from build123d import *

# Parameters (mm, degrees)
F1_DEPTH = 50.8


with BuildPart() as f1:
    # F0 (on Right) → F1 (new body)
    with BuildSketch(Plane.YZ):
        with BuildLine():
            ThreePointArc((38.1, 31.75), (36.240128, 36.240128), (31.75, 38.1))
            Line((31.75, 38.1), (12.7, 38.1))
            ThreePointArc((12.7, 38.1), (8.209872, 36.240128), (6.35, 31.75))
            Line((6.35, 31.75), (6.35, 20.128599))
            ThreePointArc((6.35, 20.128599), (6.851557, 18.393731), (8.201481, 17.194133))
            ThreePointArc((8.201481, 17.194133), (0, -19.05), (-8.201481, 17.194133))
            ThreePointArc((-8.201481, 17.194133), (-6.851557, 18.393731), (-6.35, 20.128599))
            Line((-6.35, 20.128599), (-6.35, 31.75))
            ThreePointArc((-6.35, 31.75), (-8.209872, 36.240128), (-12.7, 38.1))
            Line((-12.7, 38.1), (-31.75, 38.1))
            ThreePointArc((-31.75, 38.1), (-36.240128, 36.240128), (-38.1, 31.75))
            Line((-38.1, 31.75), (-38.1, -31.75))
            ThreePointArc((-38.1, -31.75), (-36.240128, -36.240128), (-31.75, -38.1))
            Line((-31.75, -38.1), (31.75, -38.1))
            ThreePointArc((31.75, -38.1), (36.240128, -36.240128), (38.1, -31.75))
            Line((38.1, -31.75), (38.1, 31.75))
        make_face()
    extrude(amount=F1_DEPTH)


solid = f1.part
Source: CAD feature listing. Evaluate the final solid. Frame: model axes, mm. A direction names the side the tool comes from. Round coordinates to 2 decimals unless told otherwise and drop trailing zeros. Loops run counter-clockwise (first coordinate to the right, second up) from the corner with the lowest first, then second, coordinate; pieces in that order, holes last. Notation, with made-up numbers: M -32,59 L 14,59 A9 ccw 14,65 Z; hole C -31.75,-35 d2. An arc over 180 degrees is marked long. Return JSON: item names as keys, results as strings. Group by question number.
1. Section query D-D on y = 0. Output: boundary loops of the cut face in (x, z).
2. Section query A-A on z = 0. Output: boundary loops of the cut face in (x, y), and give its area (3 significant figures).
3. Section query C-C on y = -16. Output: boundary loops of the cut face in (x, z).
4. Section query B-B on x = 22.5. Output: boundary loops of the cut face in (y, z), and give its area (3 significant figures).
5. Material intervals for line 1 along Y through (x, z) = (26, 0); line 2 along Z through (x, y) = (15, -15); line 3 along Z through (x, y) = (12, 13), sorted ascending. Write a range as from..to.
6. Pin query (flat end, axial travel): pin 1 (5 mm diameter, centred on x = 22, y = -8.5, fed in from +Z); pin 2 (12 mm diameter, centred on y = -23, z = 4, fed in from -X). Return the tip coordinate at first contact, or that it passes through.
7. Mould query, pull axis Y, two halves, no side actions, for faces 1 (the face through (25, 22, 38.1)), 2 (the face through (25, -38.1, 0)), 3 (the face through (25.04, 36.29, 36.19)), 4 (the face through (25.044, 0.719, -19.036)). Classes: released by +Y, released by -Y, zero draft, split by the parting line, or undercut.
8. Reachability of faces 5 (the face through (25.044, -6.865, 18.372)), 6 (the face through (25.04, 8.26, 36.29)), 7 (the face through (25.04, -36.19, 36.29)) from +Z, -Z, +X, -X, +Y, -Y: full face, straight path, thin tool, end or side. Return the list, or none.
Checks:
{
 "1": {"outline": "M 0,-38.1 L 50.8,-38.1 L 50.8,-19.05 L 0,-19.05 Z"},
 "2": {"outline": "M 0,-38.1 L 50.8,-38.1 L 50.8,-19.05 L 0,-19.05 Z; M 0,19.05 L 50.8,19.05 L 50.8,38.1 L 0,38.1 Z", "area": "1,940 mm²"},
 "3": {"outline": "M 0,-38.1 L 50.8,-38.1 L 50.8,-10.34 L 0,-10.34 Z; M 0,10.34 L 50.8,10.34 L 50.8,38.1 L 0,38.1 Z"},
 "4": {"outline": "M -38.1,-31.75 A6.35 ccw -31.75,-38.1 L 31.75,-38.1 A6.35 ccw 38.1,-31.75 L 38.1,31.75 A6.35 ccw 31.75,38.1 L 12.7,38.1 A6.35 ccw 6.35,31.75 L 6.35,20.13 A3.25 ccw 8.2,17.19 A19.05 cw long -8.2,17.19 A3.25 ccw -6.35,20.13 L -6.35,31.75 A6.35 ccw -12.7,38.1 L -31.75,38.1 A6.35 ccw -38.1,31.75 Z", "area": "4,370 mm²"},
 "5": {"line 1": "y = -38.1..-19.05, 19.05..38.1", "line 2": "z = -38.1..-11.74, 11.74..38.1", "line 3": "z = -38.1..-13.92, 13.92..38.1"},
 "6": {"pin 1": "stops at z = 37.87", "pin 2": "stops at x = 0"},
 "7": {"face 1": "zero draft", "face 2": "released by -Y", "face 3": "released by +Y", "face 4": "undercut"},
 "8": {"face 5": "+X, -X", "face 6": "+Z, +X, -X", "face 7": "+Z, +X, -X, -Y"}
}
